```python
from build123d import *

# Parameters (mm, degrees)
F1_R     = 2.5
F2_DEPTH = 6


with BuildPart() as f2:
    # F1 (on Front) → F2 (new body)
    with BuildSketch(Plane.XZ):
        with BuildLine():
            ThreePointArc((-48, -96.567533), (-22, -128), (-48, -159.432467))
            Line((-48, -159.432467), (-48, -191.432467))
            Line((-48, -191.432467), (48, -191.432467))
            Line((48, -191.432467), (48, -159.432467))
            ThreePointArc((48, -159.432467), (22, -128), (48, -96.567533))
            Line((48, -96.567533), (48, -31.432467))
            ThreePointArc((48, -31.432467), (22, 0), (48, 31.432467))
            Line((48, 31.432467), (48, 96.567533))
            ThreePointArc((48, 96.567533), (22, 128), (48, 159.432467))
            Line((48, 159.432467), (48, 191.432467))
            Line((48, 191.432467), (-48, 191.432467))
            Line((-48, 191.432467), (-48, 159.432467))
            ThreePointArc((-48, 159.432467), (-22, 128), (-48, 96.567533))
            Line((-48, 96.567533), (-48, 31.432467))
            ThreePointArc((-48, 31.432467), (-22, 0), (-48, -31.432467))
            Line((-48, -31.432467), (-48, -96.567533))
        make_face()
        with Locations((-38, -170.666667)):
            Circle(F1_R, mode=Mode.SUBTRACT)
        with Locations((-38, -85.333333)):
            Circle(F1_R, mode=Mode.SUBTRACT)
        with Locations((-38, -42.666667)):
            Circle(F1_R, mode=Mode.SUBTRACT)
        with Locations((38, -170.666667)):
            Circle(F1_R, mode=Mode.SUBTRACT)
        with Locations((38, -85.333333)):
            Circle(F1_R, mode=Mode.SUBTRACT)
        with Locations((38, -42.666667)):
            Circle(F1_R, mode=Mode.SUBTRACT)
        with Locations((-38, 42.666667)):
            Circle(F1_R, mode=Mode.SUBTRACT)
        with Locations((-38, 85.333333)):
            Circle(F1_R, mode=Mode.SUBTRACT)
        with Locations((-38, 170.666667)):
            Circle(F1_R, mode=Mode.SUBTRACT)
        with Locations((38, 42.666667)):
            Circle(F1_R, mode=Mode.SUBTRACT)
        with Locations((38, 85.333333)):
            Circle(F1_R, mode=Mode.SUBTRACT)
        with Locations((38, 170.666667)):
            Circle(F1_R, mode=Mode.SUBTRACT)
    extrude(amount=F2_DEPTH)


solid = f2.part
```
Input: part model. Units: mm. Frame: model coordinates. Give positions to 0.01 mm unless a question says otherwise; leave off trailing zeros. Order: outer loops, then holes, each group sorted by start corner. A loop starts at its lowest first (then second) coordinate and runs counter-clockwise, first axis right, second up.
1. Line query: probe 1 along Z at (x, y) = (26.5, -4.9); probe 2 along Z at (x, y) = (31.5, -0.3); probe 3 along X at (y, z) = (-0.5, -27.5). Output: solid intervals per line, ascending.
Computed:
probe 1: z = -191.43 to -144.36, -111.64 to -16.36, 16.36 to 111.64, 144.36 to 191.43
probe 2: z = -191.43 to -150.75, -105.25 to -22.75, 22.75 to 105.25, 150.75 to 191.43
probe 3: x = -37.64 to 37.64
2. Cut plane C-C (z = -138.5). Return loops of the section in (x, y), and give its area (3 significant figures).
Computed:
outline: (-23.77, -6) - (23.77, -6) - (23.77, 0) - (-23.77, 0) - close
area: 285 mm2
3. Draft query along Z for faces 1 (the face through (48, -3, 64)), 2 (the face through (1, -3, 191.432)), 3 (the face through (22.006, -2.958, -128.619)). Return one class per face: released by +Z, released by -Z, zero draft, split by the parting line, or undercut.
Computed:
face 1: zero draft
face 2: released by +Z
face 3: undercut
4. Cut plane A-A (x = -27.5). Return loops of the section in (y, z).
Computed:
outline: (-6, -191.43) - (0, -191.43) - (0, -145.94) - (-6, -145.94) - close; (-6, -110.06) - (0, -110.06) - (0, -17.94) - (-6, -17.94) - close; (-6, 17.94) - (0, 17.94) - (0, 110.06) - (-6, 110.06) - close; (-6, 145.94) - (0, 145.94) - (0, 191.43) - (-6, 191.43) - close
5. Cut plane B-B (y = -2.4). State how many separate pieces and enclosed holes the cut face has, and give its area (3 significant figures).
Computed:
separate pieces: 1
enclosed holes: 12
area: 29,200 mm2
